Geometry: final body of the model. Coordinates: model frame, mm. Coordinates: 2 decimals unless noted, no trailing zeros. Order: outer loops, then holes, each group sorted by start corner. A loop starts at its lowest first (then second) coordinate and runs counter-clockwise, first axis right, second up. Notation, with made-up numbers: M 11,68 L 62,68 A33 ccw 62,105 Z; hole C 39.5,53 d4. An arc over 180 degrees is marked long. One line per question, with ' | ' between items.
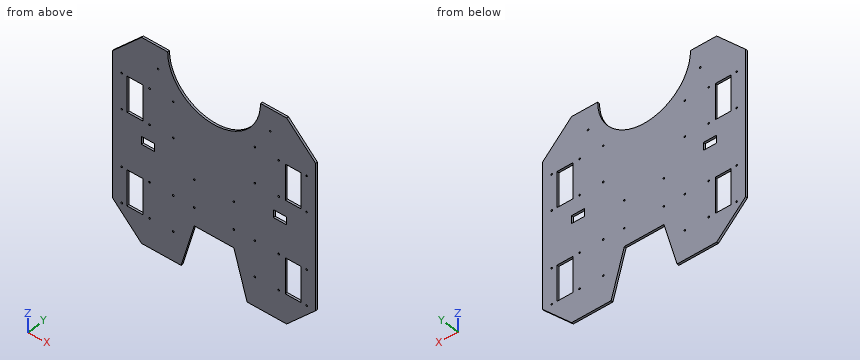
from build123d import *

# Parameters (mm, degrees)
SKETCH_1_R      = 1.55
SKETCH_1_W      = 30.4
SKETCH_1_H      = 68.58
SKETCH_1_W_2    = 25.4
SKETCH_1_H_2    = 15
EXTRUDE_1_DEPTH = 4


with BuildPart() as part:
    # 草图1 → 凸台-拉伸1 (new body)
    with BuildSketch(Plane(origin=(0, 0, 0), x_dir=(1, 0, 0), z_dir=(0, 1, 0))):
        with BuildLine():
            Line((-212.783006705, -92.69108054), (-212.783006705, 186.70891946))
            Line((-212.783006705, 186.70891946), (-156.903006705, 242.58891946))
            Line((-156.903006705, 242.58891946), (-80.703006705, 242.58891946))
            Line((-80.703006705, 242.58891946), (-55.303006705, 153.68891946))
            Line((-55.303006705, 153.68891946), (20.896993295, 153.68891946))
            Line((20.896993295, 153.68891946), (46.296993295, 242.58891946))
            Line((46.296993295, 242.58891946), (122.496993295, 242.58891946))
            Line((122.496993295, 242.58891946), (178.376993295, 186.70891946))
            Line((178.376993295, 186.70891946), (178.376993295, -92.69108054))
            Line((178.376993295, -92.69108054), (122.496993295, -148.57108054))
            Line((122.496993295, -148.57108054), (72.204993295, -148.57108054))
            ThreePointArc((72.204993295, -148.57108054), (-17.203006705, -59.16308054), (-106.611006705, -148.57108054))
            Line((-106.611006705, -148.57108054), (-156.903006705, -148.57108054))
            Line((-156.903006705, -148.57108054), (-212.783006705, -92.69108054))
        make_face()
        with Locations(Location((-141.489006705, 186.70891946, 0), (0, 0, 270))):
            Circle(SKETCH_1_R, mode=Mode.SUBTRACT)
        with Locations(Location((20.896993295, 66.00891946, 0), (0, 0, 270))):
            Circle(SKETCH_1_R, mode=Mode.SUBTRACT)
        with Locations(Location((90.746993295, -105.99108054, 0), (0, 0, 270))):
            Circle(SKETCH_1_R, mode=Mode.SUBTRACT)
        with Locations(Location((-125.153006705, -105.99108054, 0), (0, 0, 270))):
            Circle(SKETCH_1_R, mode=Mode.SUBTRACT)
        with Locations(Location((-141.489006705, 118.12891946, 0), (0, 0, 270))):
            Circle(SKETCH_1_R, mode=Mode.SUBTRACT)
        with Locations(Location((-95.769006705, 118.12891946, 0), (0, 0, 270))):
            Circle(SKETCH_1_R, mode=Mode.SUBTRACT)
        with Locations(Location((107.082993295, 118.12891946, 0), (0, 0, 270))):
            Circle(SKETCH_1_R, mode=Mode.SUBTRACT)
        with Locations(Location((-141.489006705, 8.90891946, 0), (0, 0, 270))):
            Circle(SKETCH_1_R, mode=Mode.SUBTRACT)
        with Locations(Location((61.362993295, 118.12891946, 0), (0, 0, 270))):
            Circle(SKETCH_1_R, mode=Mode.SUBTRACT)
        with Locations(Location((61.362993295, 186.70891946, 0), (0, 0, 270))):
            Circle(SKETCH_1_R, mode=Mode.SUBTRACT)
        with Locations(Location((-141.489006705, -59.67108054, 0), (0, 0, 270))):
            Circle(SKETCH_1_R, mode=Mode.SUBTRACT)
        with Locations(Location((-95.769006705, -59.67108054, 0), (0, 0, 270))):
            Circle(SKETCH_1_R, mode=Mode.SUBTRACT)
        with Locations(Location((-95.769006705, 186.70891946, 0), (0, 0, 270))):
            Circle(SKETCH_1_R, mode=Mode.SUBTRACT)
        with Locations(Location((107.082993295, -59.67108054, 0), (0, 0, 270))):
            Circle(SKETCH_1_R, mode=Mode.SUBTRACT)
        with Locations(Location((61.362993295, -59.67108054, 0), (0, 0, 270))):
            Circle(SKETCH_1_R, mode=Mode.SUBTRACT)
        with Locations(Location((107.082993295, 186.70891946, 0), (0, 0, 270))):
            Circle(SKETCH_1_R, mode=Mode.SUBTRACT)
        with Locations(Location((160.796993295, 186.70891946, 0), (0, 0, 270))):
            Circle(SKETCH_1_R, mode=Mode.SUBTRACT)
        with Locations(Location((-195.203006705, 118.12891946, 0), (0, 0, 270))):
            Circle(SKETCH_1_R, mode=Mode.SUBTRACT)
        with Locations(Location((-195.203006705, 186.70891946, 0), (0, 0, 270))):
            Circle(SKETCH_1_R, mode=Mode.SUBTRACT)
        with Locations(Location((160.796993295, 8.90891946, 0), (0, 0, 270))):
            Circle(SKETCH_1_R, mode=Mode.SUBTRACT)
        with Locations(Location((-55.303006705, 66.00891946, 0), (0, 0, 270))):
            Circle(SKETCH_1_R, mode=Mode.SUBTRACT)
        with Locations(Location((20.896993295, 119.00891946, 0), (0, 0, 270))):
            Circle(SKETCH_1_R, mode=Mode.SUBTRACT)
        with Locations(Location((-55.303006705, 119.00891946, 0), (0, 0, 270))):
            Circle(SKETCH_1_R, mode=Mode.SUBTRACT)
        with Locations(Location((160.796993295, 118.12891946, 0), (0, 0, 270))):
            Circle(SKETCH_1_R, mode=Mode.SUBTRACT)
        with Locations(Location((107.082993295, 8.90891946, 0), (0, 0, 270))):
            Circle(SKETCH_1_R, mode=Mode.SUBTRACT)
        with Locations(Location((61.362993295, 8.90891946, 0), (0, 0, 270))):
            Circle(SKETCH_1_R, mode=Mode.SUBTRACT)
        with Locations(Location((-95.769006705, 8.90891946, 0), (0, 0, 270))):
            Circle(SKETCH_1_R, mode=Mode.SUBTRACT)
        with Locations(Location((-195.203006705, 8.90891946, 0), (0, 0, 270))):
            Circle(SKETCH_1_R, mode=Mode.SUBTRACT)
        with Locations(Location((-195.203006705, -59.67108054, 0), (0, 0, 270))):
            Circle(SKETCH_1_R, mode=Mode.SUBTRACT)
        with Locations(Location((160.796993295, -59.67108054, 0), (0, 0, 270))):
            Circle(SKETCH_1_R, mode=Mode.SUBTRACT)
        with Locations((-169.563006705, -25.38108054)):
            Rectangle(SKETCH_1_W, SKETCH_1_H, mode=Mode.SUBTRACT)
        with Locations((135.156993295, 152.41891946)):
            Rectangle(SKETCH_1_W, SKETCH_1_H, mode=Mode.SUBTRACT)
        with Locations((135.156993295, -25.38108054)):
            Rectangle(SKETCH_1_W, SKETCH_1_H, mode=Mode.SUBTRACT)
        with Locations((-169.563006705, 152.41891946)):
            Rectangle(SKETCH_1_W, SKETCH_1_H, mode=Mode.SUBTRACT)
        with Locations((-144.203006705, 47.00891946)):
            Rectangle(SKETCH_1_W_2, SKETCH_1_H_2, mode=Mode.SUBTRACT)
        with Locations((109.796993295, 47.00891946)):
            Rectangle(SKETCH_1_W_2, SKETCH_1_H_2, mode=Mode.SUBTRACT)
    extrude(amount=EXTRUDE_1_DEPTH)


solid = part.part
1. Pin query (flat end, axial travel): P1, Ø1.9, axis at x = -195.2, z = -8.91, coming from the -Y side; P2, Ø2, axis at x = 135, y = 1, coming from the +Z side; P3, Ø2, axis at x = -166.5, y = 2.5, coming from the +Z side. Return the tip coordinate at first contact, or that it passes through.
Response values:
P1: passes through | P2: stops at z = 137.07 | P3: stops at z = 139.97
2. Section B-B, the plane z = 123.5. Output: boundary loops of the cut face in (x, y).
Response values:
outline: M -181.97,0 L -103.02,0 L -103.02,4 L -181.97,4 Z; M 68.62,0 L 147.57,0 L 147.57,4 L 68.62,4 Z
3. Section C-C, the plane z = -172.5. Output: boundary loops of the cut face in (x, y).
Response values:
outline: M -212.78,0 L -184.76,0 L -184.76,4 L -212.78,4 Z; M -154.36,0 L -60.68,0 L -60.68,4 L -154.36,4 Z; M 26.27,0 L 119.96,0 L 119.96,4 L 26.27,4 Z; M 150.36,0 L 178.38,0 L 178.38,4 L 150.36,4 Z
4. Section D-D, the plane y = 2.7. Give the number of separate pieces and of enclosed holes in the cut face, and give its area (3 significant figures).
Response values:
separate pieces: 1 | enclosed holes: 36 | area: 116,000 mm^2
5. Material intervals for line 1 (X direction, y = 0.9, z = -46); line 2 (X direction, y = 2.4, z = 12); line 3 (Z direction, x = -148.5, y = 3.5), sorted ascending. Write a range as [from, to].
Response values:
line 1: x = [-212.78, -156.9], [-131.5, 97.1], [122.5, 178.38] | line 2: x = [-212.78, -184.76], [-154.36, 119.96], [150.36, 178.38] | line 3: z = [-242.59, -54.51], [-39.51, 148.57]
6. Section A-A, the plane x = -164. Output: boundary loops of the cut face in (y, z).
Response values:
outline: M 0,-235.49 L 4,-235.49 L 4,-186.71 L 0,-186.71 Z; M 0,-118.13 L 4,-118.13 L 4,-8.91 L 0,-8.91 Z; M 0,59.67 L 4,59.67 L 4,141.47 L 0,141.47 Z
